from build123d import *

# Parameters (mm, degrees)
SKETCH_1_W          = 20
SKETCH_1_H          = 10
SKETCH_1_W_2        = 18
SKETCH_1_H_2        = 8
EXTRUDE_1_DEPTH     = 150
SKETCH_2_R          = 2.1
CUT_EXTRUDE_1_DEPTH = 152.657508881
SKETCH_3_R          = 5.15
SKETCH_3_R_2        = 2.1
CUT_EXTRUDE_2_DEPTH = 152.657508881


with BuildPart() as part:
    # 草图1 → 拉伸-薄壁1 (new body)
    with BuildSketch(Plane.XY):
        with Locations((10, -5)):
            Rectangle(SKETCH_1_W, SKETCH_1_H)
        with Locations((10, -5)):
            Rectangle(SKETCH_1_W_2, SKETCH_1_H_2, mode=Mode.SUBTRACT)
    extrude(amount=EXTRUDE_1_DEPTH)

    # 草图2 → 切除-拉伸1 (cut, through all)
    with BuildSketch(Plane(origin=(20, 0, 0), x_dir=(0, 0, -1), z_dir=(1, 0, 0))):
        with Locations(Location((-115, -5, 0), (0, 0, 180))):
            Circle(SKETCH_2_R)
        with Locations(Location((-125, -5, 0), (0, 0, 180))):
            Circle(SKETCH_2_R)
        Polygon((-108, -2), (-108, -8), (-100, -8), align=None)
        Polygon((-104, -2), (-96, -2), (-96, -8), align=None)
        Polygon((-90, -2), (-82, -2), (-82, -8), align=None)
        Polygon((-86, -8), (-94, -2), (-94, -8), align=None)
        Polygon((-76, -2), (-68, -2), (-68, -8), align=None)
        Polygon((-72, -8), (-80, -2), (-80, -8), align=None)
        Polygon((-62, -2), (-54, -2), (-54, -8), align=None)
        Polygon((-58, -8), (-66, -2), (-66, -8), align=None)
        Polygon((-48, -2), (-40, -2), (-40, -8), align=None)
        Polygon((-44, -8), (-52, -2), (-52, -8), align=None)
        Polygon((-34, -2), (-26, -2), (-26, -8), align=None)
        Polygon((-30, -8), (-38, -2), (-38, -8), align=None)
        Polygon((-20, -2), (-12, -2), (-12, -8), align=None)
        Polygon((-16, -8), (-24, -2), (-24, -8), align=None)
        Polygon((-139, -2), (-131, -2), (-131, -8), align=None)
        Polygon((-135, -8), (-143, -2), (-143, -8), align=None)
    extrude(amount=-CUT_EXTRUDE_1_DEPTH, mode=Mode.SUBTRACT)

    # 草图3 → 切除-拉伸2 (cut, through all)
    with BuildSketch(Plane(origin=(0, 0, 0), x_dir=(1, 0, 0), z_dir=(0, 1, 0))):
        with Locations(Location((10, -20, 0), (0, 0, 270))):
            Circle(SKETCH_3_R)
        with Locations(Location((10, -8, 0), (0, 0, 270))):
            Circle(SKETCH_3_R_2)
        with Locations(Location((10, -32, 0), (0, 0, 90))):
            Circle(SKETCH_3_R_2)
        Polygon((4, -129), (4, -145), (16, -145), align=None)
        Polygon((4, -123), (16, -123), (16, -139), align=None)
        Polygon((4, -95), (16, -95), (16, -111), align=None)
        Polygon((16, -117), (4, -101), (4, -117), align=None)
        Polygon((4, -67), (16, -67), (16, -83), align=None)
        Polygon((16, -89), (4, -73), (4, -89), align=None)
        Polygon((4, -39), (16, -39), (16, -55), align=None)
        Polygon((16, -61), (4, -45), (4, -61), align=None)
    extrude(amount=-CUT_EXTRUDE_2_DEPTH, mode=Mode.SUBTRACT)


solid = part.part
Source: CAD feature listing. Evaluate the final solid. Frame: model axes, mm. A direction names the side the tool comes from. Coordinates: 2 decimals unless noted, no trailing zeros. Loops run counter-clockwise (first coordinate to the right, second up) from the corner with the lowest first, then second, coordinate; pieces in that order, holes last. Notation, with made-up numbers: (38.5, 35) - (63.5, 35) arc R9 ccw to (63.5, 50) - close; hole circle Ø2 at (88, -7.75). An arc over 180 degrees is marked (long way). Return JSON: item names as keys, results as strings.
Q1. Access query for faces 1 (the flat face through (10.08, -0.49, 109.11)), 2 (the flat face through (10, -9.4, 150)), 3 (the flat face through (19, -5, 74)). Directions: +Z, -Z, +X, -X, +Y, -Y. A direction counts if a zero-diameter tool reaches every point of the face in a straight line with its end or side. Return the directions, or none.
Results:
{"face 1": "+Y, -Y", "face 2": "+Z, +X, -X, +Y, -Y", "face 3": "+Z, -Z"}
Q2. Material intervals for line 1 along X through (y, z) = (-5.75, 137); line 2 along X through (y, z) = (-9.25, 20); line 3 along Y through (x, z) = (17.25, 65.5), sorted ascending.
Results:
{"line 1": "0 to 1, 19 to 20", "line 2": "0 to 4.85, 15.15 to 20", "line 3": "-10 to -9, -1 to 0"}
Q3. Mould query, pull axis Y, two halves, no side actions, for faces 4 (the flat face through (10.084, -9.493, 131.112)), 5 (the flat face through (8, -9, 74)), 6 (the flat face through (0.507, -5.042, 19.944)). Classes: released by +Y, released by -Y, zero draft, split by the parting line, or undercut.
Results:
{"face 4": "zero draft", "face 5": "undercut", "face 6": "undercut"}
Q4. Contact query for flat-ended pins moving along their axis: P1, Ø8, axis at x = 17, z = 132.5, coming from the +Y side; P2, Ø1.5, axis at x = 2, y = -7, coming from the +Z side. Output: stop coordinate, or through.
Results:
{"P1": "y = 0", "P2": "through"}
Q5. Section C-C, the plane z = 32. Give the number of separate pieces and of enclosed holes in the cut face, plus the area to 3 significant figures.
Results:
{"separate pieces": "6", "enclosed holes": "0", "area": "41.6 mm2"}
Q6. Section A-A, the plane z = 141. Return loops of the section in (x, y).
Results:
{"outline": "(0, -10) - (4, -10) - (4, -9) - (1, -9) - (1, -8) - (0, -8) - close; (0, -3.5) - (1, -3.5) - (1, -1) - (4, -1) - (4, 0) - (0, 0) - close; (13, -10) - (20, -10) - (20, -8) - (19, -8) - (19, -9) - (13, -9) - close; (13, -1) - (19, -1) - (19, -3.5) - (20, -3.5) - (20, 0) - (13, 0) - close"}
Q7. Section B-B, the plane z = 8. Return loops of the section in (x, y), plus the area to 3 significant figures.
Results:
{"outline": "(0, -10) - (7.9, -10) - (7.9, -9) - (1, -9) - (1, -1) - (7.9, -1) - (7.9, 0) - (0, 0) - close; (12.1, -10) - (20, -10) - (20, 0) - (12.1, 0) - (12.1, -1) - (19, -1) - (19, -9) - (12.1, -9) - close", "area": "47.6 mm2"}
